from build123d import *

# Parameters (mm, degrees)
BOSS_EXTRUDE2_DEPTH  = 6.6
M4_CLEARANCE_HOLE2_D = 4.3


with BuildPart() as part:
    # Sketch1 → Boss-Extrude2 (new body)
    with BuildSketch(Plane(origin=(0, 0, 0), x_dir=(1, 0, 0), z_dir=(0, 1, 0))):
        with BuildLine():
            Line((5.5, 6), (-5.5, 6))
            ThreePointArc((-5.5, 6), (-4.751712409, 3.041381265), (-4.5, 0))
            ThreePointArc((-4.5, 0), (-4.751712409, -3.041381265), (-5.5, -6))
            Line((-5.5, -6), (5.5, -6))
            ThreePointArc((5.5, -6), (3.9, 0), (5.5, 6))
        make_face()
    extrude(amount=BOSS_EXTRUDE2_DEPTH)

    # M4 Clearance Hole2 (through all)
    with Locations(Plane(origin=(0, 6.6, 0), x_dir=(1, 0, 0), z_dir=(0, 1, 0))):
        with Locations((0, 0)):
            Hole(M4_CLEARANCE_HOLE2_D / 2)


solid = part.part
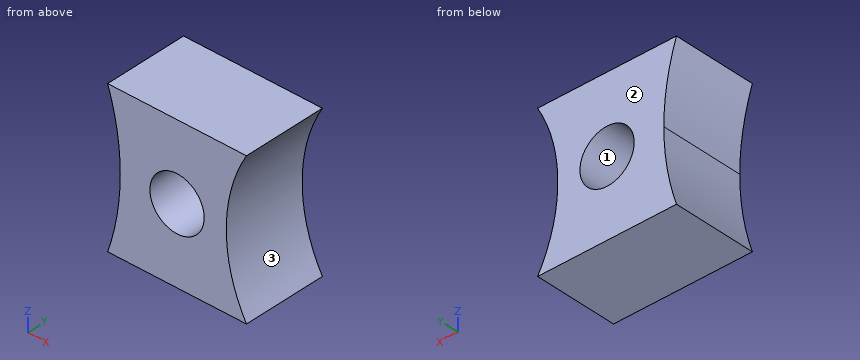
Source: CAD feature listing. Evaluate the final solid. Frame: model axes, mm. Face numbers are marked on the shaded views. Give positions to 0.01 mm unless a question says otherwise; leave off trailing zeros. Write each loop counter-clockwise with the first axis right and the second up, starting at its lowest first coordinate (ties: lowest second). Pieces come first, ordered by that corner, then holes. Notation, with made-up numbers: M 46.5,28 L 60.5,28 A23 cw 60.5,44 Z; hole C 51,-14 d3. An arc over 180 degrees is marked long. Answer as a JSON object with one key per item and string values.
Q1. Ray query, line 1 along Z through (x, y) = (0, 3.75); line 2 along Z through (x, y) = (0.75, 1); line 3 along X through (y, z) = (3, -0.5). Return the intervals inside material, ascending.
Geometry check:
{"line 1": "z = -6 to -2.15, 2.15 to 6", "line 2": "z = -6 to -2.01, 2.01 to 6", "line 3": "x = -4.51 to -2.09, 2.09 to 3.91"}
Q2. Cut plane D-D, the plane z = 5. Return the cut outline in (x, y).
Geometry check:
{"outline": "M -5.19,0 L 4.99,0 L 4.99,6.6 L -5.19,6.6 Z"}
Q3. Cut plane A-A, the plane x = 0. Return the cut outline in (y, z), then the cut area to 3 significant figures.
Geometry check:
{"outline": "M 0,-6 L 6.6,-6 L 6.6,-2.15 L 0,-2.15 Z; M 0,2.15 L 6.6,2.15 L 6.6,6 L 0,6 Z", "area": "50.8 mm^2"}
Q4. Cut plane B-B, the plane z = -0.5. Return the cut outline in (x, y).
Geometry check:
{"outline": "M -4.51,0 L -2.09,0 L -2.09,6.6 L -4.51,6.6 Z; M 2.09,0 L 3.91,0 L 3.91,6.6 L 2.09,6.6 Z"}
Q5. Mould query, pull axis X, two halves, no side actions, for the marked faces 1, 2 and 3. Classes: +X half, -X half, draft (parallel to the pull), parting line (faces both ways), or undercut.
Geometry check:
{"face 1": "undercut", "face 2": "draft", "face 3": "+X half"}
Q6. Cut plane C-C, the plane y = 0.75. Return the cut outline in (x, z), then the cut area to 3 significant figures.
Geometry check:
{"outline": "M -5.5,-6 L 5.5,-6 A12.05 cw 5.5,6 L -5.5,6 A18.5 cw Z; hole C 0,0 d4.3", "area": "96.5 mm^2"}
